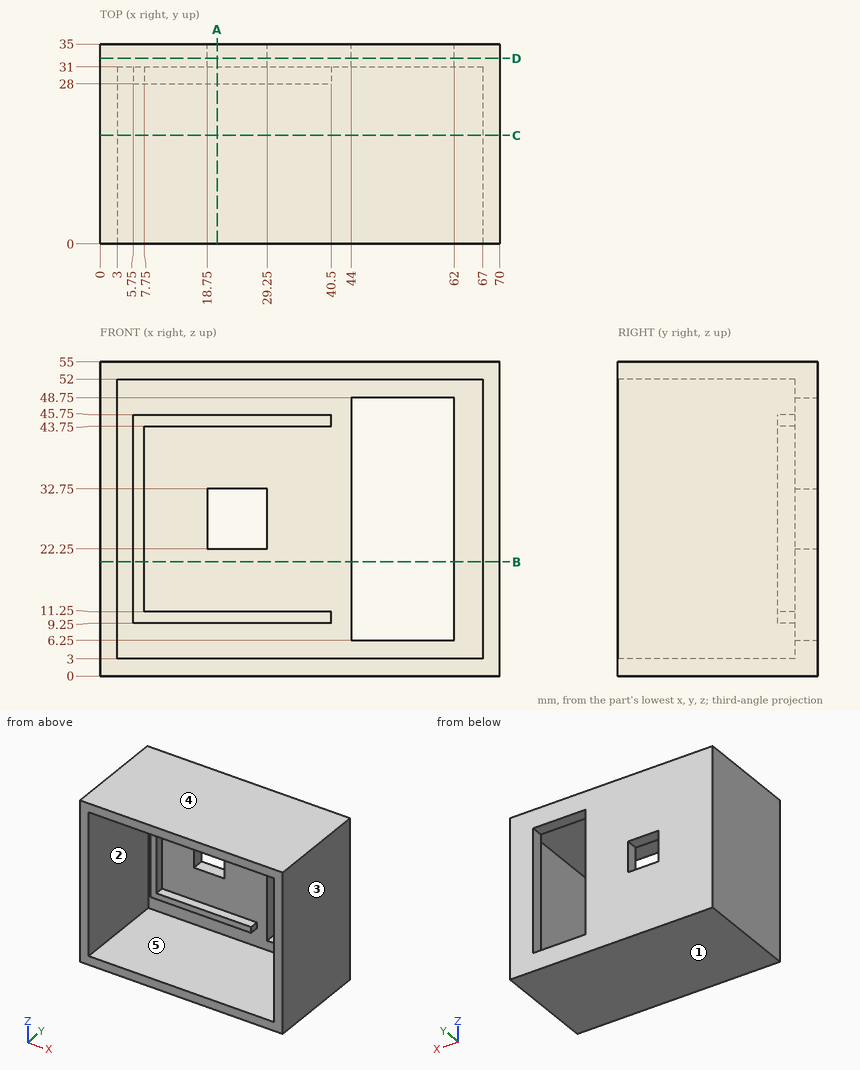
The drawing under review shows one solid part. Ordinate dimensions are in mm from its lowest x, y, z. A direction names the side the tool comes from. Round coordinates to 2 decimals unless told otherwise and drop trailing zeros. Write each loop counter-clockwise with the first axis right and the second up, starting at its lowest first coordinate (ties: lowest second). Pieces come first, ordered by that corner, then holes. Notation, with made-up numbers: M 86,-22.5 L 138,-22.5 A26 cw 138,-4.5 Z; hole C 71,43 d6. An arc over 180 degrees is marked long. One line per item, written item: value. Start each with the question number.
(1) Machinability: for the marked faces 1 and 2, which of the approach directions +Z, -Z, +X, -X, +Y, -Y give a long, thin tool a straight path to every point of the face, cutting with its end or side? Answer none if there is none.
(2) The part is to be moulded in two halves that separate along X. For the marked faces 3, 4 and 5, say which applies: released by +X, released by -X, zero draft, split by the parting line, or undercut.
(3) We need section B-B (z = 20). Give the boundary of the cut face in (x, y), and give its area (3 significant figures).
(4) We need section A-A (x = 20.5). Give the boundary of the cut face in (y, z), and give its area (3 significant figures).
(5) Insertion check: pin 1 (10.5 mm diameter, centred on x = 14.5, z = 35, fed in from -Y). The pin has a flat end and moves straight along its axis. Give the tip position at first contact, or say it passes through.
(6) We need section C-C (y = 19). Give the boundary of the cut face in (x, z), and give its area (3 significant figures).
(7) Wall thickness on line 1 (Z direction, x = 30, y = 29); line 2 (X direction, y = 21, z = 14); line 3 (Z direction, x = 46, y = 4): over which ranges is each line inside the solid? List them lowest first.
(8) We need section D-D (y = 32.5). Give the boundary of the cut face in (x, z).
Result:
1. face 1: -Z, +X, -X, +Y, -Y
1. face 2: -Y
2. face 3: released by +X
2. face 4: zero draft
2. face 5: undercut
3. outline: M 0,0 L 3,0 L 3,31 L 5.75,31 L 5.75,28 L 7.75,28 L 7.75,31 L 44,31 L 44,35 L 0,35 Z; M 62,31 L 67,31 L 67,0 L 70,0 L 70,35 L 62,35 Z
3. area: 400 mm²
4. outline: M 0,0 L 35,0 L 35,22.25 L 31,22.25 L 31,11.25 L 28,11.25 L 28,9.25 L 31,9.25 L 31,3 L 0,3 Z; M 0,52 L 31,52 L 31,45.75 L 28,45.75 L 28,43.75 L 31,43.75 L 31,32.75 L 35,32.75 L 35,55 L 0,55 Z
4. area: 376 mm²
5. pin 1: y = 31
6. outline: M 0,0 L 70,0 L 70,55 L 0,55 Z; hole M 3,3 L 67,3 L 67,52 L 3,52 Z
6. area: 714 mm²
7. line 1: 0 to 3, 9.25 to 11.25, 43.75 to 45.75, 52 to 55
7. line 2: 0 to 3, 67 to 70
7. line 3: 0 to 3, 52 to 55
8. outline: M 0,0 L 70,0 L 70,55 L 0,55 Z; hole M 18.75,22.25 L 29.25,22.25 L 29.25,32.75 L 18.75,32.75 Z; hole M 44,6.25 L 62,6.25 L 62,48.75 L 44,48.75 Z
